Input: part model. Units: mm. Frame: model coordinates. A direction names the side the tool comes from. Coordinates: 2 decimals unless noted, no trailing zeros. Write each loop counter-clockwise with the first axis right and the second up, starting at its lowest first coordinate (ties: lowest second). Pieces come first, ordered by that corner, then holes. Notation, with made-up numbers: M 72.5,15.25 L 96.5,15.25 A20 ccw 96.5,27.25 Z; hole C -25.5,-26 d1. An arc over 180 degrees is marked long. Use one line per item in the form item = value.
from build123d import *

# Parameters (mm, degrees)
SKETCH8_R                      = 12.7
BOSS_EXTRUDE6_DEPTH            = 5.08
SKETCH9_R                      = 5.969
BOSS_EXTRUDE7_DEPTH            = 4.318
F_4_40_TAPPED_HOLE1_D          = 2.2606
CIRPATTERN1_COUNT              = 6
SKETCH12_R                     = 3
CUT_EXTRUDE2_DEPTH             = 21.270727762
SKETCH13_W                     = 1.1303
SKETCH13_H                     = 12.7
F_4_40_TAPPED_HOLE2_AT_2_COUNT = 2
F_4_40_TAPPED_HOLE2_AT_2_PITCH = 4.699


with BuildPart() as part:
    # Sketch8 → Boss-Extrude6 (new body)
    with BuildSketch(Plane(origin=(0, 0, 0), x_dir=(1, 0, 0), z_dir=(0, 1, 0))):
        with Locations(Location((0, 0, 0), (0, 0, 270))):
            Circle(SKETCH8_R)
    extrude(amount=BOSS_EXTRUDE6_DEPTH)

    # Sketch9 → Boss-Extrude7 (add)
    with BuildSketch(Plane(origin=(0, 5.08, 0), x_dir=(1, 0, 0), z_dir=(0, 1, 0))):
        with Locations(Location((0, 0, 0), (0, 0, 270))):
            Circle(SKETCH9_R)
    extrude(amount=BOSS_EXTRUDE7_DEPTH)

    # #4-40 Tapped Hole1 (through all)
    with Locations(Plane(origin=(0, 5.08, 0), x_dir=(1, 0, 0), z_dir=(0, 1, 0))):
        with Locations((0, 9.3345)):
            f_4_40_tapped_hole1 = Hole(F_4_40_TAPPED_HOLE1_D / 2)

    # CirPattern1: #4-40 Tapped Hole1 ×6 about axis
    cirpattern1_axis = Axis((0, 0, 0), (0, 1, 0))
    for i in range(1, CIRPATTERN1_COUNT):
        add(f_4_40_tapped_hole1.rotate(cirpattern1_axis, i * 360 / CIRPATTERN1_COUNT), mode=Mode.SUBTRACT)

    # Sketch12 → Cut-Extrude2 (cut, through all)
    with BuildSketch(Plane(origin=(0, 9.398, 0), x_dir=(1, 0, 0), z_dir=(0, 1, 0))):
        with Locations(Location((0, 0, 0), (0, 0, 270))):
            Circle(SKETCH12_R)
    extrude(amount=-CUT_EXTRUDE2_DEPTH, mode=Mode.SUBTRACT)

    # Sketch13 → #4-40 Tapped Hole2 (revolve, cut)
    with BuildSketch(Plane.ZX.offset(7.239)):
        with Locations((0.56515, 6.35)):
            Rectangle(SKETCH13_W, SKETCH13_H)
    f_4_40_tapped_hole2 = revolve(axis=Axis((-6.35, 7.239, 0), (1, 0, 0)), mode=Mode.SUBTRACT)

    # #4-40 Tapped Hole2 at 2: #4-40 Tapped Hole2 ×2
    with Locations(*[(0, -i * F_4_40_TAPPED_HOLE2_AT_2_PITCH, 0) for i in range(1, F_4_40_TAPPED_HOLE2_AT_2_COUNT)]):
        add(f_4_40_tapped_hole2, mode=Mode.SUBTRACT)


solid = part.part
(1) Section query B-B on z = 0. Return the cut outline in (x, y), plus the area to 3 significant figures.
Computed:
outline = M -12.7,0 L -3,0 L -3,9.4 L -5.97,9.4 L -5.97,5.08 L -12.7,5.08 Z; M 3,0 L 12.7,0 L 12.7,1.41 L 3,1.41 Z; M 3,3.67 L 12.7,3.67 L 12.7,5.08 L 5.97,5.08 L 5.97,6.11 L 3,6.11 Z; M 3,8.37 L 5.97,8.37 L 5.97,9.4 L 3,9.4 Z
area = 95.6 mm^2
(2) Line query: probe 1 along X at (y, z) = (1.25, -5.5); probe 2 along Y at (x, z) = (10.25, 0); probe 3 along X at (y, z) = (2.75, 9). Output: solid intervals per line, ascending.
Computed:
probe_1 = -11.45 to -8.85, -7.32 to 7.32, 8.85 to 11.45
probe_2 = 0 to 1.41, 3.67 to 5.08
probe_3 = -8.96 to -1.08, 1.08 to 8.96
(3) First-contact query: pin 1 Ø1 at (x, y) = (9.5, 5) entering from -Z; pin 2 Ø3 at (y, z) = (7.239, 0) entering from +X; pin 3 Ø1.5 at (x, y) = (6.5, 4) entering from +Z. Flat tips, straight axial feed; report the tip coordinate or a pass-through.
Computed:
pin_1 = -8.96
pin_2 = 5.97
pin_3 = 11.32
(4) Section query D-D on z = 4.75. Return the cut outline in (x, y), plus the area to 3 significant figures.
Computed:
outline = M -11.78,0 L -9.21,0 L -9.21,5.08 L -11.78,5.08 Z; M -6.96,0 L 6.96,0 L 6.96,5.08 L 3.61,5.08 L 3.61,9.4 L -3.61,9.4 L -3.61,5.08 L -6.96,5.08 Z; M 9.21,0 L 11.78,0 L 11.78,5.08 L 9.21,5.08 Z
area = 128 mm^2
(5) Pull-direction query (Y, two-part tool) for faces 1 (the cylindrical face through (-9.162, 2.504, 4.328)), 2 (the cylindrical face through (7.81, 1.59, 0.61)), 3 (the flat face through (-5.5, 5.08, -3)); classes: pulls with the +Y half, pulls with the -Y half, needs draft (parallel to the pull), parting line crosses it, or undercut.
Computed:
face_1 = needs draft
face_2 = undercut
face_3 = pulls with the +Y half
(6) Section query C-C on y = 4. Return the cut outline in (x, z).
Computed:
outline = C 0,0 d25.4; hole C -8.08,-4.67 d2.26; hole C -8.08,4.67 d2.26; hole C 0,0 d6; hole C 0,-9.33 d2.26; hole C 0,9.33 d2.26; hole C 8.08,-4.67 d2.26; hole C 8.08,4.67 d2.26
(7) Section query A-A on x = 0. Return the cut outline in (y, z).
Computed:
outline = M 0,-12.7 L 5.08,-12.7 L 5.08,-10.46 L 0,-10.46 Z; M 0,-8.2 L 5.08,-8.2 L 5.08,-5.97 L 9.4,-5.97 L 9.4,-3 L 0,-3 Z; M 0,3 L 9.4,3 L 9.4,5.97 L 5.08,5.97 L 5.08,8.2 L 0,8.2 Z; M 0,10.46 L 5.08,10.46 L 5.08,12.7 L 0,12.7 Z
(8) Set-up query: faces 4 (the cylindrical face through (4.4, 6.9, 1.08)), 5 (the flat face through (-3, 0, 3)), 6 (the cylindrical face through (-5.3, 7.21, 2.75)). Return all of +Z, -Z, +X, -X, +Y, -Y with unobstructed straight access to the full face (end or side cutting, diameter ignored); none if empty.
Computed:
face_4 = +X
face_5 = +Z, -Z, +X, -X, -Y
face_6 = +Y
